Here's the drawing with two shaded views (mm, measured from the low corner). I have some questions. A direction names the side the tool comes from. Give positions to 0.01 mm unless a question says otherwise; leave off trailing zeros. Loops run counter-clockwise (first coordinate to the right, second up) from the corner with the lowest first, then second, coordinate; pieces in that order, holes last.
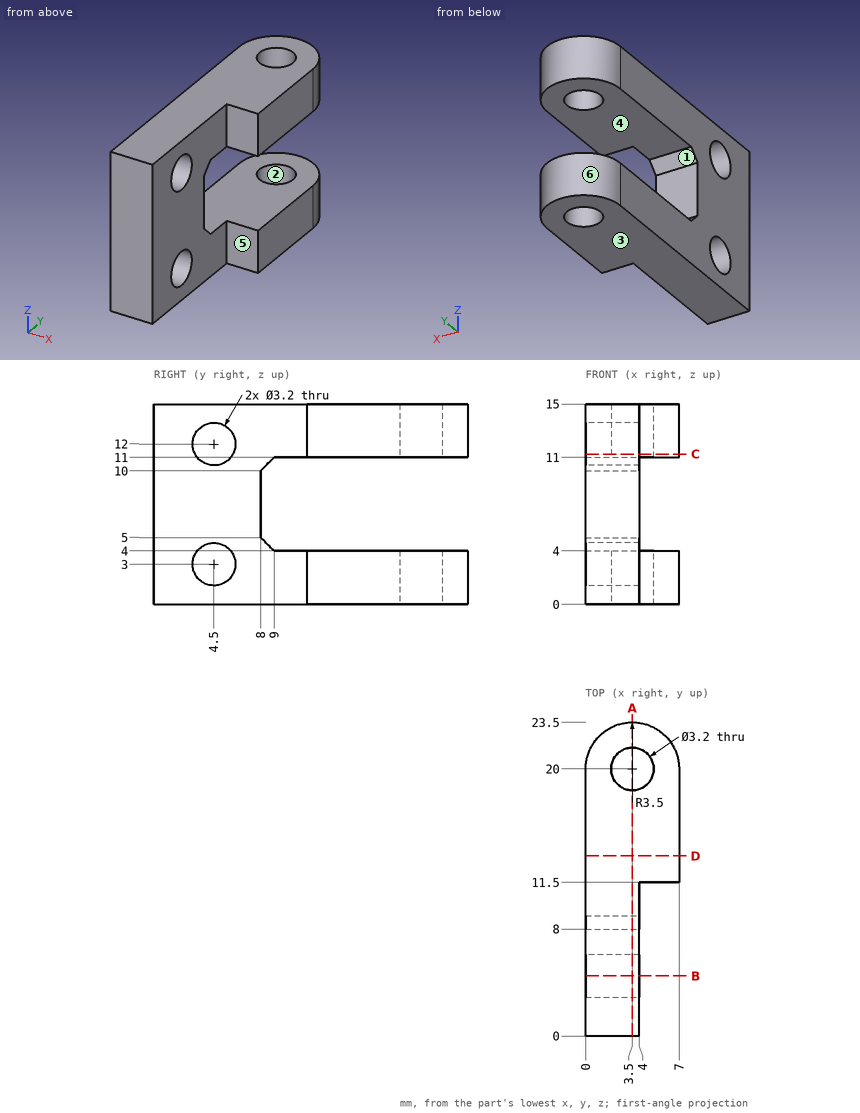
(1) Suppose I cut it at C-C on z = 11.25. List the corners of the cut face in (x, y) for me, plus the area to 3 significant figures.
Returned:
outline: (0, 0) - (4, 0) - (4, 3.09) - (0, 3.09) - close; (0, 5.91) - (4, 5.91) - (4, 11.5) - (7, 11.5) - (7, 20) arc R3.5 ccw to (0, 20) - close; hole circle Ø3.2 at (3.5, 20)
area: 105 mm2
(2) Suppose I cut it at D-D on y = 13.5. List the corners of the cut face in (x, z) for me.
Returned:
outline: (0, 0) - (7, 0) - (7, 4) - (0, 4) - close; (0, 11) - (7, 11) - (7, 15) - (0, 15) - close
(3) Suppose I cut it at A-A on x = 3.5. List the corners of the cut face in (y, z) for me, plus the area to 3 significant figures.
Returned:
outline: (0, 0) - (18.4, 0) - (18.4, 4) - (9, 4) - (8, 5) - (8, 10) - (9, 11) - (18.4, 11) - (18.4, 15) - (0, 15) - close; (21.6, 0) - (23.5, 0) - (23.5, 4) - (21.6, 4) - close; (21.6, 11) - (23.5, 11) - (23.5, 15) - (21.6, 15) - close; hole circle Ø3.2 at (4.5, 3); hole circle Ø3.2 at (4.5, 12)
area: 203 mm2
(4) Which directions (+Z, -Z, +X, -X, +Y, -Y) give clear straight access to the entire face, cutting with the end or side of a thin tool? Please do the marked faces 4, 5 and 6.
Returned:
face 4: +X, -X, +Y
face 5: +Z, -Z, +X, -Y
face 6: +Z, -Z, +Y
(5) Please list where these lines run through material, in increasing order: probe 1 along Z at (x, y) = (1.55, 4.5); probe 2 along Z at (x, y) = (0.5, 14.25); probe 3 along Z at (x, y) = (1.5, 3.25).
Returned:
probe 1: z = 0 to 1.4, 4.6 to 10.4, 13.6 to 15
probe 2: z = 0 to 4, 11 to 15
probe 3: z = 0 to 2, 4 to 11, 13 to 15
(6) Will these pins go through, and if not, where does the flat tip stop? P1, Ø8, axis at y = 10.5, z = 5.5, coming from the -X side; P2, Ø1.5, axis at x = 5, z = 2.5, coming from the -Y side; P3, Ø3.5, axis at y = 6, z = 9, coming from the +X side.
Returned:
P1: stops at x = 0
P2: stops at y = 11.5
P3: stops at x = 4
(7) Suppose I cut it at B-B on y = 4.5. List the corners of the cut face in (x, z) for me, plus the area to 3 significant figures.
Returned:
outline: (0, 0) - (4, 0) - (4, 1.4) - (0, 1.4) - close; (0, 4.6) - (4, 4.6) - (4, 10.4) - (0, 10.4) - close; (0, 13.6) - (4, 13.6) - (4, 15) - (0, 15) - close
area: 34.4 mm2
(8) Thinking about a two-plate mould opening in Z: for the marked faces 1, 2 and 3, which applies, pulls with the +Z half, pulls with the -Z half, needs draft (parallel to the pull), parting line crosses it, or undercut?
Returned:
face 1: undercut
face 2: needs draft
face 3: pulls with the -Z half
